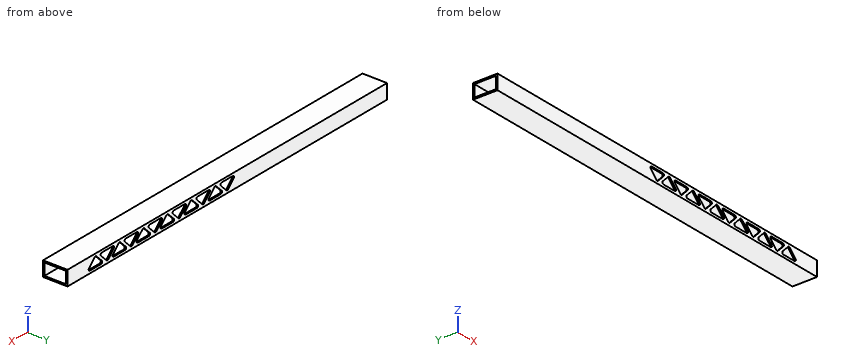
from build123d import *

# Parameters (mm, degrees)
SKETCH_W            = 25
SKETCH_H            = 15
SKETCH_W_2          = 22
SKETCH_H_2          = 12
PAD_DEPTH           = 200
POCKET_DEPTH        = 25.001
LINEARPATTERN_COUNT = 6
LINEARPATTERN_PITCH = 30


with BuildPart() as part:
    # Sketch → Pad (new body, symmetric)
    with BuildSketch(Plane.YZ):
        Rectangle(SKETCH_W, SKETCH_H)
        Rectangle(SKETCH_W_2, SKETCH_H_2, mode=Mode.SUBTRACT)
    extrude(amount=PAD_DEPTH, both=True)

    # Sketch001 (on Face4 of Pad) → Pocket (cut, through all)
    with BuildSketch(Plane(origin=(0, -12.5, 0), x_dir=(0, 0, -1), z_dir=(0, -1, 0))):
        with BuildLine():
            Line((-5, 7), (-5, -7))
            ThreePointArc((-5, -7), (-4.074025, -8.385819), (-2.43934, -8.06066))
            Line((4.56066, -1.06066), (-2.43934, -8.06066))
            ThreePointArc((4.56066, -1.06066), (5, 0), (4.56066, 1.06066))
            Line((4.56066, 1.06066), (-2.43934, 8.06066))
            ThreePointArc((-2.43934, 8.06066), (-4.074025, 8.385819), (-5, 7))
        make_face()
        with BuildLine():
            Line((-4.56066, 13.93934), (2.43934, 6.93934))
            ThreePointArc((2.43934, 6.93934), (4.074025, 6.614181), (5, 8))
            Line((5, 22), (5, 8))
            ThreePointArc((5, 22), (4.074025, 23.385819), (2.43934, 23.06066))
            Line((2.43934, 23.06066), (-4.56066, 16.06066))
            ThreePointArc((-4.56066, 16.06066), (-5, 15), (-4.56066, 13.93934))
        make_face()
    pocket = extrude(amount=-POCKET_DEPTH, mode=Mode.SUBTRACT)

    # LinearPattern: Pocket ×6
    with Locations(*[(i * LINEARPATTERN_PITCH, 0, 0) for i in range(1, LINEARPATTERN_COUNT)]):
        add(pocket, mode=Mode.SUBTRACT)


solid = part.part
Design review of the part built by this model. Coordinates are the model's own, in mm. Round coordinates to 2 decimals unless told otherwise and drop trailing zeros. Order: outer loops, then holes, each group sorted by start corner. A loop starts at its lowest first (then second) coordinate and runs counter-clockwise, first axis right, second up.
1) Consider section A-A (y = 4.5). State the section outline as (x, z) points, plus the area to 3 significant figures.
The answers:
outline: (-200, -7.5) - (200, -7.5) - (200, -6) - (-200, -6) - close; (-200, 6) - (200, 6) - (200, 7.5) - (-200, 7.5) - close
area: 1,200 mm2
2) Clearance check with a flat-ended pin moving along its axis: pin 1 Ø4 at (y, z) = (4.5, -5.5) entering from -X. State where the tip first meets the part, or that it passes through.
The answers:
pin 1: stops at x = -200
3) For L1, parallel to Z at x = -164, y = 1; L2, parallel to Y at x = -54, z = -4.5, list the stretches that pass through material, from the lowest coordinate up.
The answers:
L1: z = -7.5 to -6, 6 to 7.5
L2: y = -12.5 to -11, 11 to 12.5
4) Consider section B-B (x = -156.5). State the section outline as (y, z) points, plus the area to 3 significant figures.
The answers:
outline: (-12.5, -7.5) - (12.5, -7.5) - (12.5, 7.5) - (-12.5, 7.5) - close; hole (-11, -6) - (11, -6) - (11, 6) - (-11, 6) - close
area: 111 mm2
